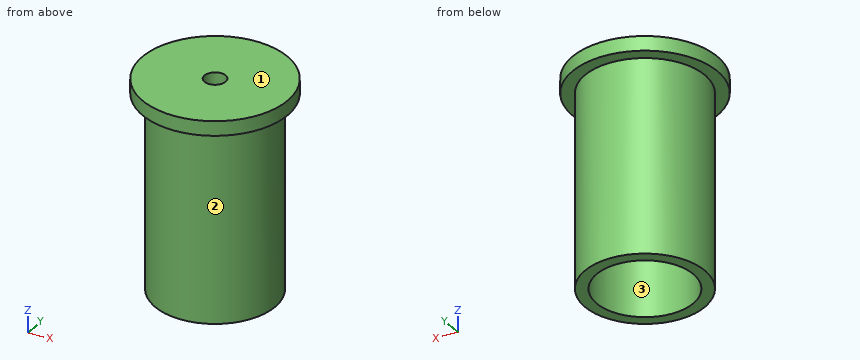
```python
from build123d import *

# Parameters (mm, degrees)
F0_R     = 15.748
F0_R_2   = 12.7
F1_DEPTH = 50.8
F2_R     = 19.05
F3_DEPTH = 3.81
F4_D     = 5.55625


with BuildPart() as f1:
    # F0 (on Top) → F1 (new body)
    with BuildSketch(Plane.XY):
        Circle(F0_R)
        Circle(F0_R_2, mode=Mode.SUBTRACT)
    extrude(amount=F1_DEPTH)

    # F2 (on face) → F3 (join)
    with BuildSketch(Plane.XY.offset(50.8)):
        Circle(F2_R)
    extrude(amount=F3_DEPTH)

    # F4 (through all)
    with Locations(Plane(origin=(0, 0, 50.8), x_dir=(1, 0, 0), z_dir=(0, 0, -1))):
        with Locations((0, 0)):
            Hole(F4_D / 2)


solid = f1.part
```
Design review of the part built by this model. Coordinates are the model's own, in mm. Face numbers are marked on the shaded views. Coordinates: 2 decimals unless noted, no trailing zeros. Loops run counter-clockwise (first coordinate to the right, second up) from the corner with the lowest first, then second, coordinate; pieces in that order, holes last. Notation, with made-up numbers: M 35,58 L 72,58 A30 cw 72,93 Z; hole C -7.75,65 d5. An arc over 180 degrees is marked long. One line per question, with ' | ' between items.
(1) We need section D-D (x = -10). Give the boundary of the cut face in (y, z), and give its area (3 significant figures).
Filled in:
outline: M -16.21,50.8 L -12.17,50.8 L -12.17,0 L -7.83,0 L -7.83,50.8 L 7.83,50.8 L 7.83,0 L 12.17,0 L 12.17,50.8 L 16.21,50.8 L 16.21,54.61 L -16.21,54.61 Z | area: 564 mm^2
(2) We need section A-A (y = 0). Give the boundary of the cut face in (x, z), and give its area (3 significant figures).
Filled in:
outline: M -19.05,50.8 L -15.75,50.8 L -15.75,0 L -12.7,0 L -12.7,50.8 L -2.78,50.8 L -2.78,54.61 L -19.05,54.61 Z; M 2.78,50.8 L 12.7,50.8 L 12.7,0 L 15.75,0 L 15.75,50.8 L 19.05,50.8 L 19.05,54.61 L 2.78,54.61 Z | area: 434 mm^2
(3) For pin 1 Ø10 at (x, z) = (-6, 41) entering from -Y; pin 2 Ø8 at (y, z) = (11, 8.5) entering from +X; pin 3 Ø1.5 at (y, z) = (-6.5, 7) entering from +X, all flat-tipped, find the tip position at first contact; note any pin that passes through.
Filled in:
pin 1: stops at y = -15.72 | pin 2: stops at x = 14.11 | pin 3: stops at x = 14.66
(4) We need section C-C (z = 45). Give the boundary of the cut face in (x, y), and give its area (3 significant figures).
Filled in:
outline: C 0,0 d31.5; hole C 0,0 d25.4 | area: 272 mm^2
(5) Wall thickness on probe 1 along Y at (x, z) = (0, 52.1); probe 2 along Z at (x, y) = (7.5, 15); probe 3 along Y at (x, z) = (0, 33): over which ranges is each line inside the solid? List them lowest first.
Filled in:
probe 1: y = -19.05 to -2.78, 2.78 to 19.05 | probe 2: z = 50.8 to 54.61 | probe 3: y = -15.75 to -12.7, 12.7 to 15.75
(6) Draft analysis for pull direction X (two halves, no side actions). For the marked faces 1, 2 and 3, state which applies: released by +X, released by -X, zero draft, split by the parting line, or undercut.
Filled in:
face 1: zero draft | face 2: split by the parting line | face 3: undercut
